```python
from build123d import *

# Parameters (mm, degrees)
SKETCH5_R          = 0.75
CUT_EXTRUDE1_DEPTH = 43.452915094
CIRPATTERN2_COUNT  = 6
SKETCH6_R          = 0.75
CUT_EXTRUDE2_DEPTH = 43.452915094
SKETCH7_R          = 2.6
CUT_EXTRUDE3_DEPTH = 4
CHAMFER1_SIZE      = 0.5
CHAMFER2_SIZE      = 1


with BuildPart() as part:
    # Sketch1 → Revolve1 (revolve)
    with BuildSketch(Plane.XY, mode=Mode.PRIVATE) as revolve1_sk:
        Polygon((10.2, 18.5), (10.2, 14.5), (8.2, 14.5), (8.2, 0), (0, 0), (0, 23.5), (25, 23.5), (25, 18.5), align=None)
    revolve(revolve1_sk.sketch.rotate(Axis((0, 0, 0), (0, 1, 0)), 90), axis=Axis((0, 0, 0), (0, 1, 0)))

    # Sketch5 → Cut-Extrude1 (cut, through all)
    with BuildSketch(Plane(origin=(0, 23.5, 0), x_dir=(1, 0, 0), z_dir=(0, 1, 0))):
        with Locations(Location((0, 21, 0), (0, 0, 270))):
            Circle(SKETCH5_R)
    cut_extrude1 = extrude(amount=-CUT_EXTRUDE1_DEPTH, mode=Mode.SUBTRACT)

    # CirPattern2: Cut-Extrude1 ×6 about axis
    cirpattern2_axis = Axis((0, 0, 0), (0, 1, 0))
    for i in range(1, CIRPATTERN2_COUNT):
        add(cut_extrude1.rotate(cirpattern2_axis, i * 360 / CIRPATTERN2_COUNT), mode=Mode.SUBTRACT)

    # Sketch6 → Cut-Extrude2 (cut, through all)
    with BuildSketch(Plane(origin=(0, 23.5, 0), x_dir=(1, 0, 0), z_dir=(0, 1, 0))):
        with Locations(Location((-10, 15, 0), (0, 0, 270))):
            Circle(SKETCH6_R)
        with Locations(Location((10, 15, 0), (0, 0, 270))):
            Circle(SKETCH6_R)
        with Locations(Location((-10, -15, 0), (0, 0, 270))):
            Circle(SKETCH6_R)
        with Locations(Location((10, -15, 0), (0, 0, 270))):
            Circle(SKETCH6_R)
    extrude(amount=-CUT_EXTRUDE2_DEPTH, mode=Mode.SUBTRACT)

    # Sketch7 → Cut-Extrude3 (cut)
    with BuildSketch(Plane.XZ):
        with Locations(Location((0, 0, 0), (0, 0, 270))):
            Circle(SKETCH7_R)
    extrude(amount=-CUT_EXTRUDE3_DEPTH, mode=Mode.SUBTRACT)

    # Sketch8 → Cut-Revolve1 (revolve, cut)
    with BuildSketch(Plane.XY, mode=Mode.PRIVATE) as cut_revolve1_sk:
        Polygon((-8.2, 5.1), (-7.7, 3.233974596), (-7.7, 0), (-8.2, 0), align=None)
    revolve(cut_revolve1_sk.sketch.rotate(Axis((0, 14.5, 0), (0, -1, 0)), 270), axis=Axis((0, 14.5, 0), (0, -1, 0)), mode=Mode.SUBTRACT)

    # Chamfer1
    chamfer1_edges = [part.edges().sort_by_distance(p)[0] for p in [
        (0, 0, 2.6),
    ]]
    chamfer(chamfer1_edges, length=CHAMFER1_SIZE)

    # Chamfer2
    chamfer2_edges = [part.edges().sort_by_distance(p)[0] for p in [
        (0, 0, -7.7),
    ]]
    chamfer(chamfer2_edges, length=CHAMFER2_SIZE)


solid = part.part
```
CAD build for the part. Positions are in the model's coordinates, mm. A direction names the side the tool comes from. Coordinates: 2 decimals unless noted, no trailing zeros. Loops run counter-clockwise (first coordinate to the right, second up) from the corner with the lowest first, then second, coordinate; pieces in that order, holes last. Notation, with made-up numbers: (-38.75, 44.5) - (-18.75, 44.5) arc R29 ccw to (-18.75, 72.5) - close; hole circle Ø10 at (-34.5, -5.5). An arc over 180 degrees is marked (long way). Use CSV: the item, a comma, the result in double quotes. Start each with the question number.
Q1. Cut at D-D, the plane y = 2.25. List the corners of the cut face in (x, z), then the cut area to 3 significant figures.
Q2. Cut at A-A, the plane x = 0. State how many separate pieces and enclosed holes the cut face has, then the cut area to 3 significant figures.
Q3. Probe probe 1 along X at (y, z) = (20.8, 10.5); probe 2 along X at (y, z) = (19.85, -15); probe 3 along Y at (x, z) = (16.5, 15). List the from-to ranges inside material, lowest first. Write a range as from..to.
Q4. Two-plate mould, pull along X, no slides. Class faces 1 (the flat face through (0, 4, 0)), 2 (the flat face through (11, 18.5, 0)), 3 (the cylindrical face through (-8.13, 9.73, 1.07)): +X half, -X half, draft (parallel to the pull), parting line (faces both ways), or undercut.
Q5. 3-axis set-ups, long thin cutter, end or side, ignore diameter. For faces 4 (the cylindrical face through (10.51, 21.04, 14.45)), 5 (the flat face through (-5, 14.5, 7)): which of +Z, -Z, +X, -X, +Y, -Y reach the whole face in a straight line?
Q6. Drop flat-ended pins along their axis: P1, Ø4, axis at x = 16.5, z = -15, coming from the -Y side; P2, Ø10, axis at y = 10, z = -15.5, coming from the +X side; P3, Ø1, axis at x = 1.5, y = 11.5, coming from the -Z side; P4, Ø12, axis at x = -13, y = 4.5, coming from the +Z side. Give the stop position or say it passes through.
Q7. Cut at C-C, the plane z = -21. List the corners of the cut face in (x, y).
Q8. Cut at B-B, the plane z = -15. List the corners of the cut face in (x, y), then the cut area to 3 significant figures.
Here are the results:
1,outline,"circle Ø15.4 at (0, 0); hole circle Ø5.2 at (0, 0)"
1,area,"165 mm2"
2,separate pieces,"3"
2,enclosed holes,"0"
2,area,"528 mm2"
3,probe 1,"-22.69..-18.94, -17.44..17.44, 18.94..22.69"
3,probe 2,"-20..-10.75, -9.25..9.25, 10.75..20"
3,probe 3,"18.5..23.5"
4,face 1,"undercut"
4,face 2,"draft"
4,face 3,"parting line"
5,face 4,"+Y, -Y"
5,face 5,"-Y"
6,P1,"y = 18.5"
6,P2,"through"
6,P3,"z = -8.14"
6,P4,"z = 4.22"
7,outline,"(-13.56, 18.5) - (-0.75, 18.5) - (-0.75, 23.5) - (-13.56, 23.5) - close; (0.75, 18.5) - (13.56, 18.5) - (13.56, 23.5) - (0.75, 23.5) - close"
8,outline,"(-20, 18.5) - (-10.75, 18.5) - (-10.75, 23.5) - (-20, 23.5) - close; (-9.25, 18.5) - (9.25, 18.5) - (9.25, 23.5) - (-9.25, 23.5) - close; (10.75, 18.5) - (20, 18.5) - (20, 23.5) - (10.75, 23.5) - close"
8,area,"185 mm2"
